Geometry check sheet. Reference: the model listing, model coordinates, mm. A direction names the side the tool comes from. Coordinates: 2 decimals unless noted, no trailing zeros. Write each loop counter-clockwise with the first axis right and the second up, starting at its lowest first coordinate (ties: lowest second). Pieces come first, ordered by that corner, then holes. Notation, with made-up numbers: (-39.5, 16) -> (2.5, 16) arc R25 cw to (2.5, 30) -> close; hole circle Ø7 at (63, 85). An arc over 180 degrees is marked (long way). Answer in a Markdown table with one row per item. Add a question column.
1. Depth check by flat-ended pin: P1, Ø1, axis at x = 120, z = -70.5, coming from the +Y side; P2, Ø1, axis at x = 41.5, z = -7, coming from the -Y side; P3, Ø1, axis at x = 154, z = 36.5, coming from the +Y side. Enter the tip coordinate at first touch or a pass-through.
2. Cross-section at C-C on z = 69. Record the cut outline in (x, y).
3. Cross-section at A-A on x = 102.5. Record the cut outline in (y, z).
4. Mould release check, pull along Z, two halves, no side actions. Record for faces 1 (the cylindrical face through (87.655, 250.205, 7.883)), 2 (the flat face through (177.8, 134, 18)), 3 (the flat face through (88, 34, 0)): pulls with the +Z half, pulls with the -Z half, needs draft (parallel to the pull), parting line crosses it, or undercut.
5. Cross-section at B-B on y = 18.5. Record the cut outline in (x, z).
6. Scan lines: L1, parallel to Z at x = 89.5, y = 34; L2, parallel to Z at x = 162.5, y = 78.5; L3, parallel to Y at x = 144, z = 17. Record each from-to range of solid material in increasing order. Write a range as from..to.
7. Set-up check for faces 4 (the flat face through (88, 137, 78.74)), 5 (the flat face through (88, 34, 78.74)), 6 (the flat face through (90.145, 253.877, -15.675)), 7 (the flat face through (0, 134, 18)): record each of +Z, -Z, +X, -X, +Y, -Y from which the full face is reachable in a straight line by a thin tool's end or side.
```python
from build123d import *

# Parameters (mm, degrees)
BOSS_EXTRUDE1_DEPTH = 177.8
BOSS_EXTRUDE2_DEPTH = 177.8


with BuildPart() as part:
    # Sketch2 → Boss-Extrude1 (new body)
    with BuildSketch(Plane(origin=(0, 0, 0), x_dir=(0, 0, -1), z_dir=(1, 0, 0))):
        with BuildLine():
            Line((9.446959598, 242.605367243), (76.143806671, 205.754714731))
            Line((76.143806671, 205.754714731), (0.427641882, 68.714279363))
            ThreePointArc((0.427641882, 68.714279363), (0.108631196, 67.912266317), (0, 67.056))
            Line((0, 67.056), (0, 0))
            Line((0, 0), (-78.74, 0))
            Line((-78.74, 0), (-78.74, 69.342))
            ThreePointArc((-78.74, 69.342), (-79.215672983, 71.084383578), (-80.510720637, 72.343358118))
            Line((-80.510720637, 72.343358118), (-83.662355749, 74.084666973))
            Line((-83.662355749, 74.084666973), (-78.74, 82.993752329))
            Line((-78.74, 82.993752329), (-78.74, 192.532))
            ThreePointArc((-78.74, 192.532), (-63.696886188, 233.267747455), (-25.788612916, 254.449324625))
            ThreePointArc((-25.788612916, 254.449324625), (-7.634921788, 250.121653844), (9.446959598, 242.605367243))
        make_face()
    extrude(amount=BOSS_EXTRUDE1_DEPTH)

    # Sketch3 → Boss-Extrude2 (add)
    with BuildSketch(Plane(origin=(177.8, 0, 0), x_dir=(0, 0, -1), z_dir=(1, 0, 0))):
        Polygon((76.143806671, 205.754714731), (88.427357508, 227.986997088), (21.730510436, 264.8376496), (9.446959598, 242.605367243), align=None)
    extrude(amount=-BOSS_EXTRUDE2_DEPTH)


solid = part.part
```
Results found:
| question | item | result |
|---|---|---|
| 1 | P1 | stops at y = 238.17 |
| 1 | P2 | stops at y = 79.7 |
| 1 | P3 | stops at y = 251.95 |
| 2 | outline | (0, 0) -> (177.8, 0) -> (177.8, 226.09) -> (0, 226.09) -> close |
| 3 | outline | (0, 0) -> (67.06, 0) arc R3.43 cw to (68.71, -0.43) -> (227.99, -88.43) -> (264.84, -21.73) -> (242.61, -9.45) arc R103.54 ccw to (254.45, 25.79) arc R62.68 ccw to (192.53, 78.74) -> (82.99, 78.74) -> (74.08, 83.66) -> (72.34, 80.51) arc R3.43 cw to (69.34, 78.74) -> (0, 78.74) -> close |
| 4 | face 1 | undercut |
| 4 | face 2 | needs draft |
| 4 | face 3 | pulls with the -Z half |
| 5 | outline | (0, 0) -> (177.8, 0) -> (177.8, 78.74) -> (0, 78.74) -> close |
| 6 | L1 | z = 0..78.74 |
| 6 | L2 | z = -5.83..81.22 |
| 6 | L3 | y = 0..252.79 |
| 7 | face 4 | +Z, +X, -X, +Y |
| 7 | face 5 | +Z, +X, -X, -Y |
| 7 | face 6 | +X, -X, +Y |
| 7 | face 7 | +Z, -Z, -X, +Y, -Y |
